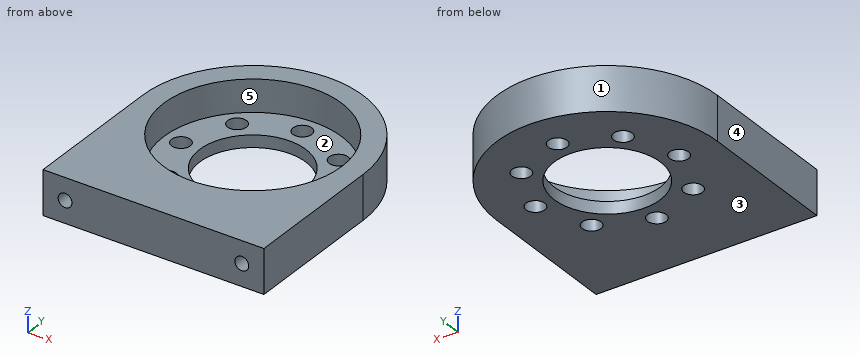
```python
from build123d import *

# Parameters (mm, degrees)
ESQUISSE1_R             = 9.6
BOSS_EXTRU_1_DEPTH      = 8
ESQUISSE2_R             = 16.1
ENL_V_MAT_EXTRU_1_DEPTH = 5.8
ENL_V_MAT_EXTRU_2_REACH = 10
ESQUISSE3_R             = 1.7
ESQUISSE4_R             = 1.25
ENL_V_MAT_EXTRU_3_DEPTH = 15


with BuildPart() as part:
    # Esquisse1 → Boss.-Extru.1 (new body)
    with BuildSketch(Plane.XY):
        with BuildLine():
            Line((-20, 0), (-20, -26))
            Line((-20, -26), (20, -26))
            Line((20, -26), (20, 0))
            ThreePointArc((20, 0), (0, 20), (-20, 0))
        make_face()
        Circle(ESQUISSE1_R, mode=Mode.SUBTRACT)
    extrude(amount=BOSS_EXTRU_1_DEPTH)

    # Esquisse2 → Enlèv. mat.-Extru.1 (cut)
    with BuildSketch(Plane.XY.offset(8)):
        Circle(ESQUISSE2_R)
    extrude(amount=-ENL_V_MAT_EXTRU_1_DEPTH, mode=Mode.SUBTRACT)

    # Esquisse3 → Enlèv. mat.-Extru.2 (cut, up to next)
    with BuildSketch(Plane(origin=(0, 0, 0), x_dir=(-1, 0, 0), z_dir=(0, 0, -1)), mode=Mode.PRIVATE) as enl_v_mat_extru_2_sk1:
        with Locations((0, 13)):
            Circle(ESQUISSE3_R)
    enl_v_mat_extru_2_tool1 = extrude(enl_v_mat_extru_2_sk1.sketch, amount=-ENL_V_MAT_EXTRU_2_REACH, mode=Mode.PRIVATE) & part.part
    add(enl_v_mat_extru_2_tool1.solids().sort_by_distance((0, 13, 0))[0], mode=Mode.SUBTRACT)
    # Esquisse3 → Enlèv. mat.-Extru.2 (cut, up to next)
    with BuildSketch(Plane(origin=(0, 0, 0), x_dir=(-1, 0, 0), z_dir=(0, 0, -1)), mode=Mode.PRIVATE) as enl_v_mat_extru_2_sk2:
        with Locations((9.192388155, 9.192388155)):
            Circle(ESQUISSE3_R)
    enl_v_mat_extru_2_tool2 = extrude(enl_v_mat_extru_2_sk2.sketch, amount=-ENL_V_MAT_EXTRU_2_REACH, mode=Mode.PRIVATE) & part.part
    add(enl_v_mat_extru_2_tool2.solids().sort_by_distance((-9.192388, 9.192388, 0))[0], mode=Mode.SUBTRACT)
    # Esquisse3 → Enlèv. mat.-Extru.2 (cut, up to next)
    with BuildSketch(Plane(origin=(0, 0, 0), x_dir=(-1, 0, 0), z_dir=(0, 0, -1)), mode=Mode.PRIVATE) as enl_v_mat_extru_2_sk3:
        with Locations((13, 0)):
            Circle(ESQUISSE3_R)
    enl_v_mat_extru_2_tool3 = extrude(enl_v_mat_extru_2_sk3.sketch, amount=-ENL_V_MAT_EXTRU_2_REACH, mode=Mode.PRIVATE) & part.part
    add(enl_v_mat_extru_2_tool3.solids().sort_by_distance((-13, 0, 0))[0], mode=Mode.SUBTRACT)
    # Esquisse3 → Enlèv. mat.-Extru.2 (cut, up to next)
    with BuildSketch(Plane(origin=(0, 0, 0), x_dir=(-1, 0, 0), z_dir=(0, 0, -1)), mode=Mode.PRIVATE) as enl_v_mat_extru_2_sk4:
        with Locations((9.192388155, -9.192388155)):
            Circle(ESQUISSE3_R)
    enl_v_mat_extru_2_tool4 = extrude(enl_v_mat_extru_2_sk4.sketch, amount=-ENL_V_MAT_EXTRU_2_REACH, mode=Mode.PRIVATE) & part.part
    add(enl_v_mat_extru_2_tool4.solids().sort_by_distance((-9.192388, -9.192388, 0))[0], mode=Mode.SUBTRACT)
    # Esquisse3 → Enlèv. mat.-Extru.2 (cut, up to next)
    with BuildSketch(Plane(origin=(0, 0, 0), x_dir=(-1, 0, 0), z_dir=(0, 0, -1)), mode=Mode.PRIVATE) as enl_v_mat_extru_2_sk5:
        with Locations((0, -13)):
            Circle(ESQUISSE3_R)
    enl_v_mat_extru_2_tool5 = extrude(enl_v_mat_extru_2_sk5.sketch, amount=-ENL_V_MAT_EXTRU_2_REACH, mode=Mode.PRIVATE) & part.part
    add(enl_v_mat_extru_2_tool5.solids().sort_by_distance((0, -13, 0))[0], mode=Mode.SUBTRACT)
    # Esquisse3 → Enlèv. mat.-Extru.2 (cut, up to next)
    with BuildSketch(Plane(origin=(0, 0, 0), x_dir=(-1, 0, 0), z_dir=(0, 0, -1)), mode=Mode.PRIVATE) as enl_v_mat_extru_2_sk6:
        with Locations((-9.192388155, -9.192388155)):
            Circle(ESQUISSE3_R)
    enl_v_mat_extru_2_tool6 = extrude(enl_v_mat_extru_2_sk6.sketch, amount=-ENL_V_MAT_EXTRU_2_REACH, mode=Mode.PRIVATE) & part.part
    add(enl_v_mat_extru_2_tool6.solids().sort_by_distance((9.192388, -9.192388, 0))[0], mode=Mode.SUBTRACT)
    # Esquisse3 → Enlèv. mat.-Extru.2 (cut, up to next)
    with BuildSketch(Plane(origin=(0, 0, 0), x_dir=(-1, 0, 0), z_dir=(0, 0, -1)), mode=Mode.PRIVATE) as enl_v_mat_extru_2_sk7:
        with Locations((-13, 0)):
            Circle(ESQUISSE3_R)
    enl_v_mat_extru_2_tool7 = extrude(enl_v_mat_extru_2_sk7.sketch, amount=-ENL_V_MAT_EXTRU_2_REACH, mode=Mode.PRIVATE) & part.part
    add(enl_v_mat_extru_2_tool7.solids().sort_by_distance((13, 0, 0))[0], mode=Mode.SUBTRACT)
    # Esquisse3 → Enlèv. mat.-Extru.2 (cut, up to next)
    with BuildSketch(Plane(origin=(0, 0, 0), x_dir=(-1, 0, 0), z_dir=(0, 0, -1)), mode=Mode.PRIVATE) as enl_v_mat_extru_2_sk8:
        with Locations((-9.192388155, 9.192388155)):
            Circle(ESQUISSE3_R)
    enl_v_mat_extru_2_tool8 = extrude(enl_v_mat_extru_2_sk8.sketch, amount=-ENL_V_MAT_EXTRU_2_REACH, mode=Mode.PRIVATE) & part.part
    add(enl_v_mat_extru_2_tool8.solids().sort_by_distance((9.192388, 9.192388, 0))[0], mode=Mode.SUBTRACT)

    # Esquisse4 → Enlèv. mat.-Extru.3 (cut)
    with BuildSketch(Plane.XZ.offset(26)):
        with Locations((-16, 4)):
            Circle(ESQUISSE4_R)
        with Locations((16, 4)):
            Circle(ESQUISSE4_R)
    extrude(amount=-ENL_V_MAT_EXTRU_3_DEPTH, mode=Mode.SUBTRACT)


solid = part.part
```
CAD build for the part. Positions are in the model's coordinates, mm. Face numbers are marked on the shaded views. A direction names the side the tool comes from. Give positions to 0.01 mm unless a question says otherwise; leave off trailing zeros. Write each loop counter-clockwise with the first axis right and the second up, starting at its lowest first coordinate (ties: lowest second). Pieces come first, ordered by that corner, then holes. Notation, with made-up numbers: (-28, 51.25) -> (26, 51.25) arc R4 ccw to (26, 56.25) -> close; hole circle Ø8 at (36.25, -24). An arc over 180 degrees is marked (long way). Write each question's results on one line, items separated by ' | '.
1. Cut at D-D, the plane x = 0. Write the cut outline in (y, z), then the cut area to 3 significant figures.
Geometry check:
outline: (-26, 0) -> (-14.7, 0) -> (-14.7, 2.2) -> (-16.1, 2.2) -> (-16.1, 8) -> (-26, 8) -> close; (-11.3, 0) -> (-9.6, 0) -> (-9.6, 2.2) -> (-11.3, 2.2) -> close; (9.6, 0) -> (11.3, 0) -> (11.3, 2.2) -> (9.6, 2.2) -> close; (14.7, 0) -> (20, 0) -> (20, 8) -> (16.1, 8) -> (16.1, 2.2) -> (14.7, 2.2) -> close | area: 124 mm²
2. Drop flat-ended pins along their axis: P1, Ø3, axis at x = 9.19, y = 9.19, coming from the -Z side; P2, Ø16, axis at x = 7, y = 7, coming from the +Z side; P3, Ø2, axis at x = 16, z = 4, coming from the -Y side; P4, Ø4, axis at x = 0, y = -13, coming from the +Z side. Give the stop position or say it passes through.
Geometry check:
P1: through | P2: z = 8 | P3: y = -11 | P4: z = 2.2
3. Two-plate mould, pull along Y, no slides. Class the marked faces 1, 2 and 3: pulls with the +Y half, pulls with the -Y half, needs draft (parallel to the pull), parting line crosses it, or undercut.
Geometry check:
face 1: pulls with the +Y half | face 2: undercut | face 3: needs draft
4. Cut at C-C, the plane y = -13. Write the cut outline in (x, z), then the cut area to 3 significant figures.
Geometry check:
outline: (-20, 0) -> (-1.7, 0) -> (-1.7, 2.2) -> (-9.5, 2.2) -> (-9.5, 8) -> (-20, 8) -> close; (1.7, 0) -> (20, 0) -> (20, 8) -> (9.5, 8) -> (9.5, 2.2) -> (1.7, 2.2) -> close; hole circle Ø2.5 at (-16, 4); hole circle Ø2.5 at (16, 4) | area: 193 mm²
5. Wall check: probe 1 along Y at (x, z) = (0, 0.95); probe 2 along Y at (x, z) = (1, 1); probe 3 along Z at (x, y) = (-16, -15.25). Give the ranges that are in metal, low to high. Write a range as [from, to].
Geometry check:
probe 1: [-26, -14.7], [-11.3, -9.6], [9.6, 11.3], [14.7, 20] | probe 2: [-26, -14.37], [-11.63, -9.55], [9.55, 11.63], [14.37, 19.97] | probe 3: [0, 2.75], [5.25, 8]
6. Cut at B-B, the plane x = -13. Write the cut outline in (y, z).
Geometry check:
outline: (-26, 0) -> (-1.7, 0) -> (-1.7, 2.2) -> (-9.5, 2.2) -> (-9.5, 8) -> (-26, 8) -> close; (1.7, 0) -> (15.2, 0) -> (15.2, 8) -> (9.5, 8) -> (9.5, 2.2) -> (1.7, 2.2) -> close
7. Which spindle directions (+Z, -Z, +X, -X, +Y, -Y) get a long thin tool onto all of the face, cutting with end or side? Do the marked faces 4 and 5. Say none if no direction does.
Geometry check:
face 4: +Z, -Z, -X, +Y, -Y | face 5: +Z
8. Cut at A-A, the plane z = 4. Write the cut outline in (x, y).
Geometry check:
outline: (-20, -26) -> (-17.25, -26) -> (-17.25, -11) -> (-14.75, -11) -> (-14.75, -26) -> (14.75, -26) -> (14.75, -11) -> (17.25, -11) -> (17.25, -26) -> (20, -26) -> (20, 0) arc R20 ccw to (-20, 0) -> close; hole circle Ø32.2 at (0, 0)
